from build123d import *

# Parameters (mm, degrees)
F0_R     = 1
F1_DEPTH = 1.5
F2_R     = 6
F3_DEPTH = 0.5


with BuildPart() as f1:
    # F0 (on Top) → F1 (new body)
    with BuildSketch(Plane.XY):
        with BuildLine():
            Line((13.461538, 1.946017), (1.153846, 4.865043))
            ThreePointArc((1.153846, 4.865043), (0, 5), (-1.153846, 4.865043))
            Line((-1.153846, 4.865043), (-13.461538, 1.946017))
            ThreePointArc((-13.461538, 1.946017), (-15, 0), (-13.461538, -1.946017))
            Line((-13.461538, -1.946017), (-1.153846, -4.865043))
            ThreePointArc((-1.153846, -4.865043), (0, -5), (1.153846, -4.865043))
            Line((1.153846, -4.865043), (13.461538, -1.946017))
            ThreePointArc((13.461538, -1.946017), (15, 0), (13.461538, 1.946017))
        make_face()
        with Locations((-13, 0)):
            Circle(F0_R, mode=Mode.SUBTRACT)
        with Locations((13, 0)):
            Circle(F0_R, mode=Mode.SUBTRACT)
    extrude(amount=F1_DEPTH)

    # F2 (on face) → F3 (cut)
    with BuildSketch(Plane.XY.offset(1.5)):
        Circle(F2_R)
    extrude(amount=-F3_DEPTH, mode=Mode.SUBTRACT)


solid = f1.part
Source: CAD feature listing. Evaluate the final solid. Frame: model axes, mm. A direction names the side the tool comes from. Coordinates: 2 decimals unless noted, no trailing zeros. Loops run counter-clockwise (first coordinate to the right, second up) from the corner with the lowest first, then second, coordinate; pieces in that order, holes last. Notation, with made-up numbers: (8.25, 74.5) - (35.25, 74.5) arc R20 ccw to (35.25, 86.5) - close; hole circle Ø9 at (-9.5, 77.5). An arc over 180 degrees is marked (long way). One line per item, written item: value. Start each with the question number.
1. Section B-B (x = 13). Return the cut outline in (y, z), and give its area (3 significant figures).
2. Section C-C (y = -2.5). Return the cut outline in (x, z).
3. Set-up query: faces 1 (the cylindrical face through (-15, 0, 1)), 2 (the flat face through (0, 0, 1)). Return all of +Z, -Z, +X, -X, +Y, -Y with unobstructed straight access to the full face (end or side cutting, diameter ignored); none if empty.
4. Section D-D (x = 1.5). Return the cut outline in (y, z), and give its area (3 significant figures).
5. Contact query for flat-ended pins moving along their axis: P1, Ø1.2, axis at x = 13, y = 0, coming from the -Z side; P2, Ø5, axis at x = -2.5, y = 2, coming from the +Z side. Output: stop coordinate, or through.
6. Section A-A (y = 0). Return the cut outline in (x, z), and give its area (3 significant figures).
7. Ray query, L1, parallel to X at y = -0.5, z = 0.8; L2, parallel to X at y = 0.75, z = 0.4; L3, parallel to Y at x = 13, z = 0.75. Return the intervals inside material, ascending.
Verdict:
1. outline: (-2.06, 0) - (-1, 0) - (-1, 1.5) - (-2.06, 1.5) - close; (1, 0) - (2.06, 0) - (2.06, 1.5) - (1, 1.5) - close
1. area: 3.17 mm2
2. outline: (-11.13, 0) - (11.13, 0) - (11.13, 1.5) - (5.45, 1.5) - (5.45, 1) - (-5.45, 1) - (-5.45, 1.5) - (-11.13, 1.5) - close
3. face 1: +Z, -Z, -X
3. face 2: +Z
4. outline: (-4.78, 0) - (4.78, 0) - (4.78, 1) - (-4.78, 1) - close
4. area: 9.57 mm2
5. P1: passes through
5. P2: stops at z = 1
6. outline: (-15, 0) - (-14, 0) - (-14, 1.5) - (-15, 1.5) - close; (-12, 0) - (12, 0) - (12, 1.5) - (6, 1.5) - (6, 1) - (-6, 1) - (-6, 1.5) - (-12, 1.5) - close; (14, 0) - (15, 0) - (15, 1.5) - (14, 1.5) - close
6. area: 33.0 mm2
7. L1: x = -14.94 to -13.87, -12.13 to 12.13, 13.87 to 14.94
7. L2: x = -14.85 to -13.66, -12.34 to 12.34, 13.66 to 14.85
7. L3: y = -2.06 to -1, 1 to 2.06
